```python
from build123d import *

# Parameters (mm, degrees)
SKETCH1_R       = 0.8
EXTRUDE9_DEPTH  = 4
SKETCH2_R       = 0.55
EXTRUDE10_DEPTH = 5
SKETCH3_R       = 0.3
EXTRUDE11_DEPTH = 10


with BuildPart() as part:
    # Sketch1 → Extrude9 (new body)
    with BuildSketch(Plane(origin=(0, 0, 0), x_dir=(1, 0, 0), z_dir=(0, 1, 0))):
        with BuildLine():
            Line((-14.4, 14.85), (-14.4, 3.15))
            Line((-14.4, 3.15), (-15.25, 3.15))
            ThreePointArc((-15.25, 3.15), (-18.4, 0), (-15.25, -3.15))
            Line((-15.25, -3.15), (-14.4, -3.15))
            Line((-14.4, -3.15), (-14.4, -14.85))
            ThreePointArc((-14.4, -14.85), (-11.25, -18), (-8.1, -14.85))
            Line((-8.1, -14.85), (-8.1, -6.725))
            ThreePointArc((-8.1, -6.725), (-5.625, -4.25), (-3.15, -6.725))
            Line((-3.15, -6.725), (-3.15, -12.7))
            ThreePointArc((-3.15, -12.7), (0, -15.85), (3.15, -12.7))
            Line((3.15, -12.7), (3.15, -6.725))
            ThreePointArc((3.15, -6.725), (5.625, -4.25), (8.1, -6.725))
            Line((8.1, -6.725), (8.1, -14.85))
            ThreePointArc((8.1, -14.85), (11.25, -18), (14.4, -14.85))
            Line((14.4, -14.85), (14.4, -3.15))
            Line((14.4, -3.15), (15.25, -3.15))
            ThreePointArc((15.25, -3.15), (18.4, 0), (15.25, 3.15))
            Line((15.25, 3.15), (14.4, 3.15))
            Line((14.4, 3.15), (14.4, 14.85))
            ThreePointArc((14.4, 14.85), (11.25, 18), (8.1, 14.85))
            Line((8.1, 14.85), (8.1, 6.725))
            ThreePointArc((8.1, 6.725), (5.625, 4.25), (3.15, 6.725))
            Line((3.15, 6.725), (3.15, 12.7))
            ThreePointArc((3.15, 12.7), (0, 15.85), (-3.15, 12.7))
            Line((-3.15, 12.7), (-3.15, 6.725))
            ThreePointArc((-3.15, 6.725), (-5.625, 4.25), (-8.1, 6.725))
            Line((-8.1, 6.725), (-8.1, 14.85))
            ThreePointArc((-8.1, 14.85), (-11.25, 18), (-14.4, 14.85))
        make_face()
        with Locations((-11.25, 14.85)):
            Circle(SKETCH1_R, mode=Mode.SUBTRACT)
        with Locations((0, 12.7)):
            Circle(SKETCH1_R, mode=Mode.SUBTRACT)
        with Locations((11.25, 14.85)):
            Circle(SKETCH1_R, mode=Mode.SUBTRACT)
        with Locations((11.25, -14.85)):
            Circle(SKETCH1_R, mode=Mode.SUBTRACT)
        with Locations((0, -12.7)):
            Circle(SKETCH1_R, mode=Mode.SUBTRACT)
        with Locations((-11.25, -14.85)):
            Circle(SKETCH1_R, mode=Mode.SUBTRACT)
    extrude(amount=EXTRUDE9_DEPTH)

    # Sketch2 → Extrude10 (cut, through all)
    with BuildSketch(Plane(origin=(0, 0, 0), x_dir=(1, 0, 0), z_dir=(0, 1, 0))):
        with Locations((13.5, 0)):
            Circle(SKETCH2_R)
        with BuildLine():
            Line((-14.35, 0.55), (-12.65, 0.55))
            ThreePointArc((-12.65, 0.55), (-12.1, 0), (-12.65, -0.55))
            Line((-12.65, -0.55), (-14.35, -0.55))
            ThreePointArc((-14.35, -0.55), (-14.9, 0), (-14.35, 0.55))
        make_face()
    extrude(amount=EXTRUDE10_DEPTH, mode=Mode.SUBTRACT)

    # Sketch3 → Extrude11 (cut)
    with BuildSketch(Plane(origin=(0, 0, 0), x_dir=(1, 0, 0), z_dir=(0, 1, 0))):
        with Locations((-3.6, 0)):
            Circle(SKETCH3_R)
        with Locations((3.6, 0)):
            Circle(SKETCH3_R)
        Circle(SKETCH3_R)
        with Locations((0, -7)):
            Circle(SKETCH3_R)
        with BuildLine():
            Line((-7.2, 0.264383356), (-6.6, 0.264383356))
            ThreePointArc((-6.6, 0.264383356), (-6.335616644, 0), (-6.6, -0.264383356))
            Line((-6.6, -0.264383356), (-7.2, -0.264383356))
            ThreePointArc((-7.2, -0.264383356), (-7.464383356, 0), (-7.2, 0.264383356))
        make_face()
        with BuildLine():
            Line((6.6, 0.264383356), (7.2, 0.264383356))
            ThreePointArc((7.2, 0.264383356), (7.464383356, 0), (7.2, -0.264383356))
            Line((7.2, -0.264383356), (6.6, -0.264383356))
            ThreePointArc((6.6, -0.264383356), (6.335616644, 0), (6.6, 0.264383356))
        make_face()
    extrude(amount=EXTRUDE11_DEPTH, mode=Mode.SUBTRACT)


solid = part.part
```
The model under review builds one solid part; all positions refer to its coordinate system, in mm. A direction names the side the tool comes from. Round coordinates to 2 decimals unless told otherwise and drop trailing zeros. Write each loop counter-clockwise with the first axis right and the second up, starting at its lowest first coordinate (ties: lowest second). Pieces come first, ordered by that corner, then holes. Notation, with made-up numbers: M 66,13 L 99,13 A15 cw 99,36 Z; hole C -34,-26.75 d8. An arc over 180 degrees is marked long. Use CSV: the item, a comma, the result in double quotes. Start each with the question number.
(1) We need section B-B, the plane x = -11.25. State the section outline as (y, z) points.
(2) We need section A-A, the plane z = 9. State the section outline as (x, y) points.
(3) The part is to be moulded in two halves that separate along X. For faces 1 (the face through (-4.3, 0, -0.3)), 2 (the face through (-8.1, 2, -11)), 3 (the face through (-14.4, 2, 9)), say which applies: +X half, -X half, draft (parallel to the pull), parting line (faces both ways), or undercut.
(4) Tool access review of faces 4 (the face through (15, 2, -3.15)), 5 (the face through (-3.15, 2, 10)), 6 (the face through (-15, 2, -3.15)), 7 (the face through (-14.9, 2, 0)), 8 (the face through (8.1, 2, -11)): name each direction out of +Z, -Z, +X, -X, +Y, -Y from which nothing blocks a thin tool from reaching the whole face with its end or side.
(5) We need section D-D, the plane x = -16. State the section outline as (y, z) points.
(6) Clearance check with flat-ended pins moving along their axes: P1, Ø2, axis at y = 2, z = 9.5, coming from the +X side; P2, Ø2, axis at y = 1, z = 6, coming from the -X side; P3, Ø1, axis at x = 11.25, z = -14.85, coming from the +Y side; P4, Ø1.9, axis at x = -14, y = 1.5, coming from the -Z side. State where each tip first meets the part, or that it passes through.
(7) For line 1 along Z through (x, y) = (0, 2.15); line 2 along Z through (x, y) = (-11.25, 1.7); line 3 along X through (y, z) = (3.4, 7.5), list the stretches that pass through material, from the lowest coordinate up.
(8) We need section C-C, the plane y = 1.6. State how many separate pieces and enclosed holes the cut face has, then the cut area to 3 significant figures.
Findings:
1,outline,"M 0,-18 L 4,-18 L 4,-15.65 L 0,-15.65 Z; M 0,-14.05 L 4,-14.05 L 4,14.05 L 0,14.05 Z; M 0,15.65 L 4,15.65 L 4,18 L 0,18 Z"
2,outline,"M -14.4,0 L -8.1,0 L -8.1,4 L -14.4,4 Z; M -3.15,0 L 3.15,0 L 3.15,4 L -3.15,4 Z; M 8.1,0 L 14.4,0 L 14.4,4 L 8.1,4 Z"
3,face 1,"draft"
3,face 2,"undercut"
3,face 3,"-X half"
4,face 4,"-Z, +X, +Y, -Y"
4,face 5,"+Z, +Y, -Y"
4,face 6,"-Z, -X, +Y, -Y"
4,face 7,"+Y, -Y"
4,face 8,"-Z, +Y, -Y"
5,outline,"M 0,-3.06 L 4,-3.06 L 4,3.06 L 0,3.06 Z"
6,P1,"x = 14.4"
6,P2,"x = -14.4"
6,P3,"through"
6,P4,"z = -17.44"
7,line 1,"-15.85 to -13.5, -11.9 to -0.3, 0.3 to 6.7, 7.3 to 11.9, 13.5 to 15.85"
7,line 2,"-18 to -15.65, -14.05 to 14.05, 15.65 to 18"
7,line 3,"-14.4 to -8.1, -3.15 to 3.15, 8.1 to 14.4"
8,separate pieces,"1"
8,enclosed holes,"14"
8,area,"746 mm^2"
